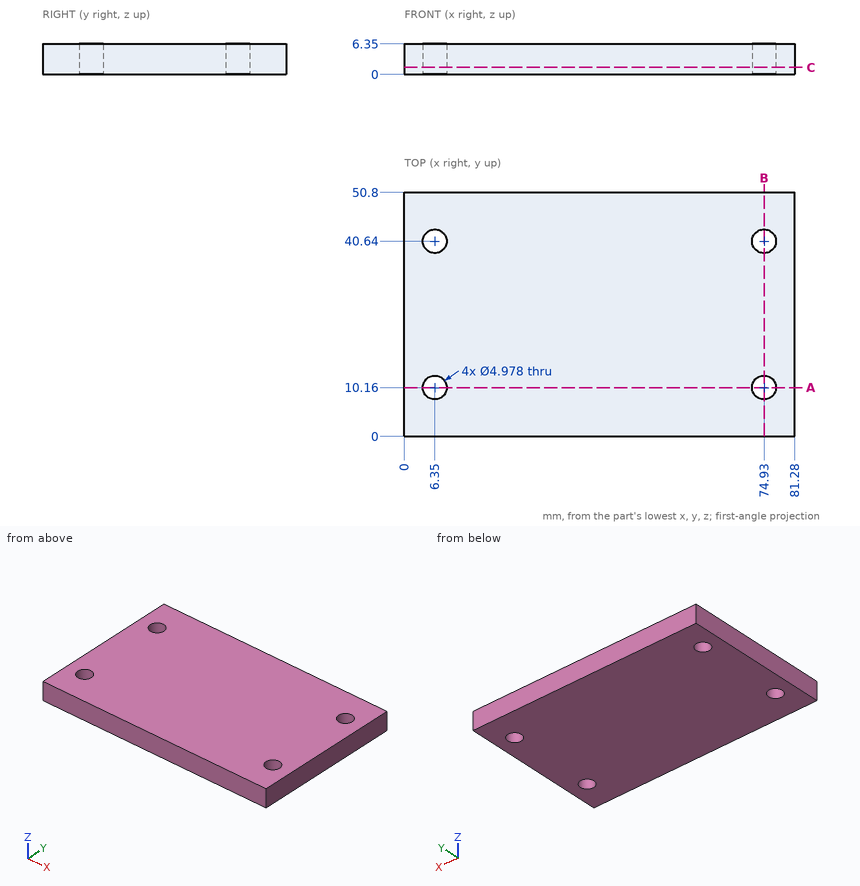
Geometry check sheet. Reference: drawing and pictorial views, mm from the part's lowest x, y, z. Give positions to 0.01 mm unless a question says otherwise; leave off trailing zeros. Order: outer loops, then holes, each group sorted by start corner. A loop starts at its lowest first (then second) coordinate and runs counter-clockwise, first axis right, second up. Notation, with made-up numbers: M 26.5,61.5 L 48.5,61.5 A14 ccw 48.5,72.5 Z; hole C 68,21.25 d6. An arc over 180 degrees is marked long. Answer in a Markdown table with one row per item.
1) Cross-section at A-A, the plane y = 10.16. Enter the section's corners in (x, z), plus the area to 3 significant figures.
Filled sheet:
| item | result |
|---|---|
| outline | M 0,0 L 3.86,0 L 3.86,6.35 L 0,6.35 Z; M 8.84,0 L 72.44,0 L 72.44,6.35 L 8.84,6.35 Z; M 77.42,0 L 81.28,0 L 81.28,6.35 L 77.42,6.35 Z |
| area | 453 mm2 |
2) Cross-section at C-C, the plane z = 1.5. Enter the section's corners in (x, y).
Filled sheet:
| item | result |
|---|---|
| outline | M 0,0 L 81.28,0 L 81.28,50.8 L 0,50.8 Z; hole C 6.35,10.16 d4.98; hole C 6.35,40.64 d4.98; hole C 74.93,10.16 d4.98; hole C 74.93,40.64 d4.98 |
3) Cross-section at B-B, the plane x = 74.93. Enter the section's corners in (y, z), plus the area to 3 significant figures.
Filled sheet:
| item | result |
|---|---|
| outline | M 0,0 L 7.67,0 L 7.67,6.35 L 0,6.35 Z; M 12.65,0 L 38.15,0 L 38.15,6.35 L 12.65,6.35 Z; M 43.13,0 L 50.8,0 L 50.8,6.35 L 43.13,6.35 Z |
| area | 259 mm2 |
4) Thickness scan on L1, parallel to Y at x = 6.35, z = 2.25. Record the ranges inside material, lowest first. Write a range as [from, to].
Filled sheet:
| item | result |
|---|---|
| L1 | y = [0, 7.67], [12.65, 38.15], [43.13, 50.8] |
